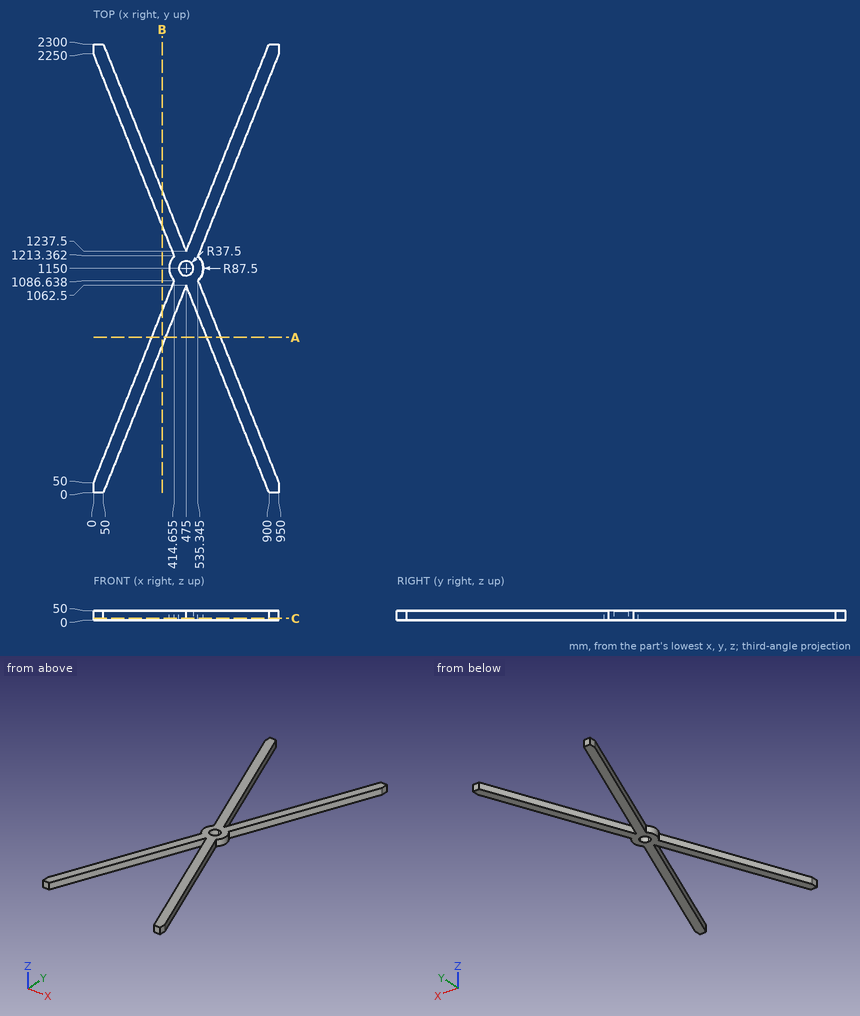
Could you check a few things on this drawing? It's one solid part, dimensions in mm from its lowest x, y, z. Give positions to 0.01 mm unless a question says otherwise; leave off trailing zeros. Order: outer loops, then holes, each group sorted by start corner. A loop starts at its lowest first (then second) coordinate and runs counter-clockwise, first axis right, second up. Notation, with made-up numbers: (-14.75, 15.25) - (3.25, 15.25) arc R17 ccw to (3.25, 35.25) - close; hole circle Ø6 at (-18, 31). An arc over 180 degrees is marked (long way). One line per question, with ' | ' between items. Start each with the question number.
Item 1: I need wall thicknesses on probe 1 along X at (y, z) = (767, 28); probe 2 along X at (y, z) = (2043, 6.5); probe 3 along Y at (x, z) = (481.5, 29.5). Which ranges of each line are inside material? Lowest first, please. Write a range as [from, to].
Item 2: I want a section at C-C on z = 10.5. Write out the boundary of the cut face in (x, y) (1 decimal).
Item 3: I'm going to push flat-ended pins straight in: pin 1 Ø4 at (y, z) = (270, 31.5) entering from +X; pin 2 Ø1.5 at (y, z) = (1530.5, 45) entering from +X; pin 3 Ø3 at (y, z) = (2008, 35) entering from -X. Where does each tip first touch, or does it pass through?
Item 4: I want a section at B-B on x = 351.5. Write out the boundary of the cut face in (y, z).
Item 5: I want a section at A-A on y = 796. Write out the boundary of the cut face in (x, z).
Verdict:
1) probe 1: [286.8, 356.8], [593.2, 663.2] | probe 2: [82.8, 152.8], [797.2, 867.2] | probe 3: [1046.25, 1113.07], [1186.93, 1253.75]
2) outline: (0, 0) - (50, 0) - (475, 1062.5) - (900, 0) - (950, 0) - (950, 50) - (535.3, 1086.6) arc R87.5 ccw to (535.3, 1213.4) - (950, 2250) - (950, 2300) - (900, 2300) - (475, 1237.5) - (50, 2300) - (0, 2300) - (0, 2250) - (414.7, 1213.4) arc R87.5 ccw to (414.7, 1086.6) - (0, 50) - close; hole circle Ø75 at (475, 1150)
3) pin 1: x = 862.8 | pin 2: x = 662.5 | pin 3: x = 96.2
4) outline: (753.75, 0) - (928.75, 0) - (928.75, 50) - (753.75, 50) - close; (1371.25, 0) - (1546.25, 0) - (1546.25, 50) - (1371.25, 50) - close
5) outline: (298.4, 0) - (368.4, 0) - (368.4, 50) - (298.4, 50) - close; (581.6, 0) - (651.6, 0) - (651.6, 50) - (581.6, 50) - close
